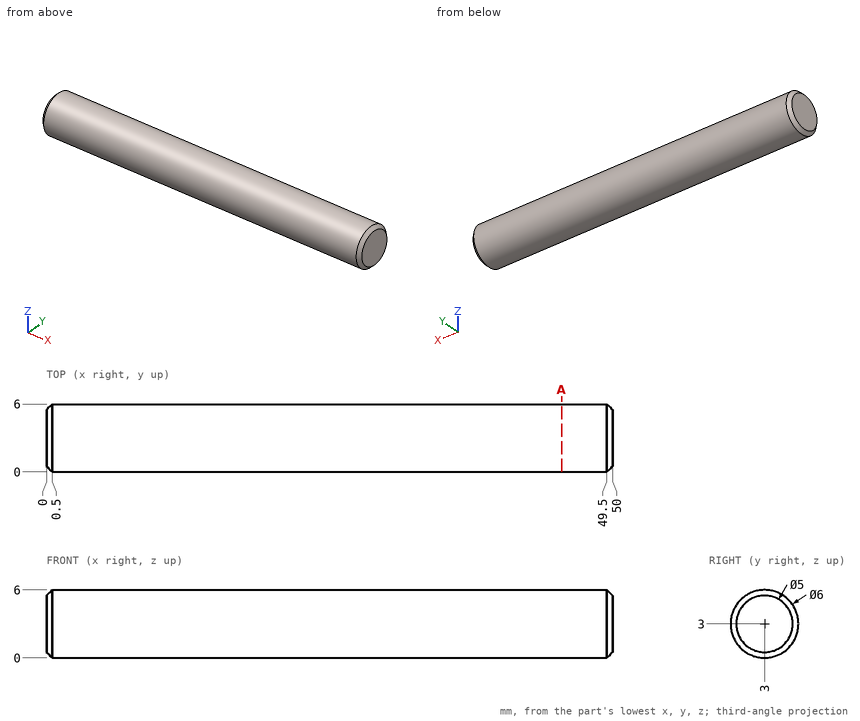
Job drawing, mm, ordinate dimensions from the low corner. One solid piece. Round coordinates to 2 decimals unless told otherwise and drop trailing zeros. Write each loop counter-clockwise with the first axis right and the second up, starting at its lowest first coordinate (ties: lowest second). Pieces come first, ordered by that corner, then holes.
1) Band-saw the part on A-A, the plane x = 45.5. List the corners of the cut face in (y, z).
2) Pin check, flat tips, straight feed: pin 1 (1 mm diameter, centred on x = 11.5, y = 4, fed in from +Z); pin 2 (1 mm diameter, centred on x = 41, y = 5.5, fed in from -Z). Stop position of each tip, or through.
3) Drill centre lines: probe 1 along Y at (x, z) = (31.5, 3.2); probe 2 along Z at (x, y) = (40.5, 4.65). Where is each one in solid material? Low to high.
Ans:
1. outline: circle Ø6 at (3, 3)
2. pin 1: stops at z = 5.96
2. pin 2: stops at z = 0.76
3. probe 1: y = 0.01 to 5.99
3. probe 2: z = 0.49 to 5.51
